Input: part model. Units: mm. Frame: model coordinates. Face numbers are marked on the shaded views. A direction names the side the tool comes from. Coordinates: 2 decimals unless noted, no trailing zeros. Order: outer loops, then holes, each group sorted by start corner. A loop starts at its lowest first (then second) coordinate and runs counter-clockwise, first axis right, second up. Notation, with made-up numbers: (5, 59) -> (59, 59) arc R15 ccw to (59, 66) -> close; hole circle Ø6 at (57, 64). An arc over 180 degrees is marked (long way). One line per item, written item: value. Start each with the question number.
from build123d import *

# Parameters (mm, degrees)
F0_W     = 100
F0_H     = 50
F1_DEPTH = 10
F2_W     = 100
F2_H     = 50
F2_W_2   = 95
F2_H_2   = 5
F2_H_3   = 14
F2_H_4   = 12
F3_DEPTH = 1


with BuildPart() as f1:
    # F0 (on Front) → F1 (new body)
    with BuildSketch(Plane.XZ):
        Rectangle(F0_W, F0_H)
    extrude(amount=F1_DEPTH)

    # F2 (on face) → F3 (join)
    with BuildSketch(Plane.XZ.offset(10)):
        Rectangle(F2_W, F2_H)
        with Locations((-0.025468, -20.277101)):
            Rectangle(F2_W_2, F2_H_2, mode=Mode.SUBTRACT)
        with Locations((-0.025468, -9.200179)):
            Rectangle(F2_W_2, F2_H_3, mode=Mode.SUBTRACT)
        with Locations((-0.025468, 9.043411)):
            Rectangle(F2_W_2, F2_H_4, mode=Mode.SUBTRACT)
        with Locations((-0.025468, 18.697258)):
            Rectangle(F2_W_2, F2_H_2, mode=Mode.SUBTRACT)
    extrude(amount=F3_DEPTH)


solid = f1.part
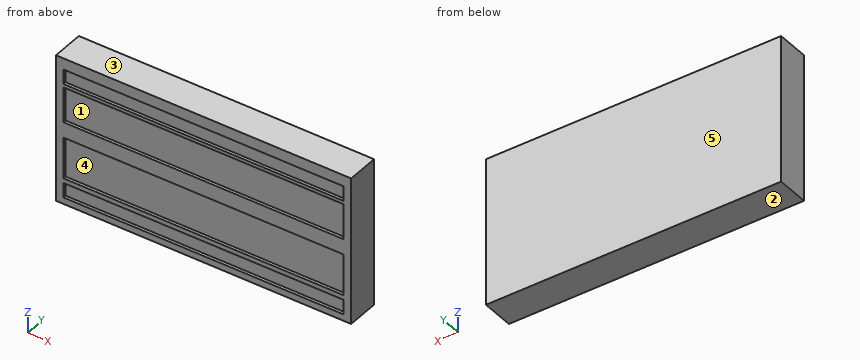
1) Section query A-A, the plane x = 2.5. Return the cut outline in (y, z), plus the area to 3 significant figures.
2) Ray query, line 1 along Z through (x, y) = (-1.5, -10.5); line 2 along Y through (x, z) = (-7, 5). Return the intervals inside material, ascending. Write a range as from..to.
3) Mould query, pull axis Z, two halves, no side actions, for the marked faces 3, 4 and 5. Classes: +Z half, -Z half, draft (parallel to the pull), parting line (faces both ways), or undercut.
4) Pin query (flat end, axial travel): pin 1 Ø3.5 at (x, z) = (7.5, 10) entering from -Y. Return the tip coordinate at first contact, or that it passes through.
5) Section query B-B, the plane z = -7.5. Return the cut outline in (x, y).
6) Access query for the marked faces 1 and 2. Directions: +Z, -Z, +X, -X, +Y, -Y. A direction counts if a zero-diameter tool reaches every point of the face in a straight line with its end or side. Return the directions, or none.
Entries:
1. outline: (-11, -25) -> (0, -25) -> (0, 25) -> (-11, 25) -> (-11, 21.2) -> (-10, 21.2) -> (-10, 16.2) -> (-11, 16.2) -> (-11, 15.04) -> (-10, 15.04) -> (-10, 3.04) -> (-11, 3.04) -> (-11, -2.2) -> (-10, -2.2) -> (-10, -16.2) -> (-11, -16.2) -> (-11, -17.78) -> (-10, -17.78) -> (-10, -22.78) -> (-11, -22.78) -> close
1. area: 514 mm2
2. line 1: z = -25..-22.78, -17.78..-16.2, -2.2..3.04, 15.04..16.2, 21.2..25
2. line 2: y = -10..0
3. face 3: +Z half
3. face 4: undercut
3. face 5: draft
4. pin 1: stops at y = -10
5. outline: (-50, -11) -> (-47.53, -11) -> (-47.53, -10) -> (47.47, -10) -> (47.47, -11) -> (50, -11) -> (50, 0) -> (-50, 0) -> close
6. face 1: -Y
6. face 2: -Z, +X, -X, +Y, -Y
